Source: CAD feature listing. Evaluate the final solid. Frame: model axes, mm. Face numbers are marked on the shaded views. A direction names the side the tool comes from. Give positions to 0.01 mm unless a question says otherwise; leave off trailing zeros. Order: outer loops, then holes, each group sorted by start corner. A loop starts at its lowest first (then second) coordinate and runs counter-clockwise, first axis right, second up. Notation, with made-up numbers: M -35.75,-36 L 10.25,-36 A31 ccw 10.25,-3 Z; hole C -11,60 d8. An arc over 180 degrees is marked long. Answer as a JSON object with one key per item and string values. Group by question number.
1. Pull-direction query (Y, two-part tool) for the marked faces 1, 2, 3 and 4; classes: +Y half, -Y half, draft (parallel to the pull), parting line (faces both ways), or undercut.
2. Section query B-B (y = 75). Output: boundary loops of the cut face in (x, z) (3 decimals), plus the area to 3 significant figures.
3. Section query D-D (x = 20). Output: boundary loops of the cut face in (y, z).
4. Material intervals for L1, parallel to Y at x = 47, z = 4.1; L2, parallel to X at y = 18.5, z = 0.3; L3, parallel to Y at x = -2.5, z = 3.15, sorted ascending. Write a range as [from, to].
5. Section query A-A (x = 47). Output: boundary loops of the cut face in (y, z) (3 decimals), plus the area to 3 significant figures.
6. Set-up query: the marked faces 5 and 6. Return all of +Z, -Z, +X, -X, +Y, -Y with unobstructed straight access to the full face (end or side cutting, diameter ignored); none if empty.
7. Section query C-C (z = 5.1). Count the separate pieces of the cut face and the enclosed holes in it, plus the area to 3 significant figures.
8. Pin query (flat end, axial travel): P1, Ø1.8, axis at x = -3, y = 75, coming from the -Z side; P2, Ø3, axis at y = 66.5, z = 4, coming from the +X side; P3, Ø1.8, axis at x = -2.5, z = 4, coming from the -Y side. Return the tip coordinate at first contact, or that it passes through.
from build123d import *

# Parameters (mm, degrees)
BOSS_EXTRU_1_DEPTH       = 6
ESQUISSE2_R              = 1.5
ENL_V_MAT_EXTRU_1_DEPTH  = 6
ESQUISSE5_R              = 1.5
ENL_V_MAT_EXTRU_6_DEPTH  = 6
ESQUISSE6_R              = 2.995
ENL_V_MAT_EXTRU_7_DEPTH  = 3
ESQUISSE9_W              = 44
ESQUISSE9_H              = 20
BOSS_EXTRU_3_DEPTH       = 6
ESQUISSE10_W             = 25
ESQUISSE10_H             = 6.5
ENL_V_MAT_EXTRU_9_DEPTH  = 4
ENL_V_MAT_EXTRU_11_DEPTH = 6


with BuildPart() as part:
    # Esquisse1 → Boss.-Extru.1 (new body)
    with BuildSketch(Plane.XY):
        Polygon((0, 80), (0, 90), (44, 90), (44, 80), (50, 80), (50, 70), (44, 70), (44, 25), (50, 25), (50, 15), (44, 15), (44, 0), (0, 0), (0, 15), (-6, 15), (-6, 25), (0, 25), (0, 70), (-6, 70), (-6, 80), align=None)
    extrude(amount=BOSS_EXTRU_1_DEPTH)

    # Esquisse2 → Enlèv. mat.-Extru.1 (cut)
    with BuildSketch(Plane.XY.offset(6)):
        with Locations((20, 85)):
            Circle(ESQUISSE2_R)
    extrude(amount=-ENL_V_MAT_EXTRU_1_DEPTH, mode=Mode.SUBTRACT)

    # Esquisse5 → Enlèv. mat.-Extru.6 (cut)
    with BuildSketch(Plane(origin=(0, 0, 0), x_dir=(-1, 0, 0), z_dir=(0, 0, -1))):
        with Locations((3, 75)):
            Circle(ESQUISSE5_R)
        with Locations((3, 20)):
            Circle(ESQUISSE5_R)
        with Locations(Location((-47, 20, 0), (0, 0, 180))):
            Circle(ESQUISSE5_R)
        with Locations(Location((-47, 75, 0), (0, 0, 180))):
            Circle(ESQUISSE5_R)
    extrude(amount=-ENL_V_MAT_EXTRU_6_DEPTH, mode=Mode.SUBTRACT)

    # Esquisse6 → Enlèv. mat.-Extru.7 (cut)
    with BuildSketch(Plane(origin=(0, 0, 0), x_dir=(-1, 0, 0), z_dir=(0, 0, -1))):
        with Locations((3, 20)):
            Circle(ESQUISSE6_R)
        with Locations((3, 75)):
            Circle(ESQUISSE6_R)
        with Locations(Location((-47, 75, 0), (0, 0, 180))):
            Circle(ESQUISSE6_R)
        with Locations(Location((-47, 20, 0), (0, 0, 180))):
            Circle(ESQUISSE6_R)
    extrude(amount=-ENL_V_MAT_EXTRU_7_DEPTH, mode=Mode.SUBTRACT)

    # Esquisse9 → Boss.-Extru.3 (add)
    with BuildSketch(Plane.XY.offset(6)):
        with Locations((22, -10)):
            Rectangle(ESQUISSE9_W, ESQUISSE9_H)
    extrude(amount=-BOSS_EXTRU_3_DEPTH)

    # Esquisse10 → Enlèv. mat.-Extru.9 (cut)
    with BuildSketch(Plane.XY.offset(6)):
        with Locations((12.5, -9.75)):
            Rectangle(ESQUISSE10_W, ESQUISSE10_H)
    extrude(amount=-ENL_V_MAT_EXTRU_9_DEPTH, mode=Mode.SUBTRACT)

    # Esquisse11 → Enlèv. mat.-Extru.11 (cut)
    with BuildSketch(Plane.XY.offset(6)):
        Polygon((29, 71.292517007), (10, -2.207482993), (15, -3.5), (34, 70), align=None)
    extrude(amount=-ENL_V_MAT_EXTRU_11_DEPTH, mode=Mode.SUBTRACT)


solid = part.part
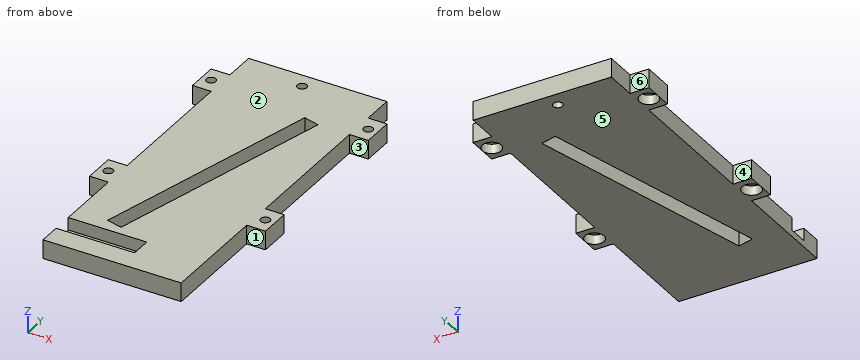
Answer sheet:
{
 "1": {"face 1": "-Y half", "face 2": "draft", "face 3": "undercut", "face 4": "undercut"},
 "2": {"outline": "M -6,0 L -5.995,0 L -5.995,3 L -4.5,3 L -4.5,6 L -6,6 Z; M -1.5,3 L -0.005,3 L -0.005,0 L 44.005,0 L 44.005,3 L 45.5,3 L 45.5,6 L -1.5,6 Z; M 48.5,3 L 49.995,3 L 49.995,0 L 50,0 L 50,6 L 48.5,6 Z", "area": "282 mm^2"},
 "3": {"outline": "M -20,0 L 15.84,0 L 15.84,6 L -6.5,6 L -6.5,2 L -13,2 L -13,6 L -20,6 Z; M 36.48,0 L 83.5,0 L 83.5,6 L 36.48,6 Z; M 86.5,0 L 90,0 L 90,6 L 86.5,6 Z"},
 "4": {"L1": "[15, 18.5], [21.5, 25], [70, 73.5], [76.5, 80]", "L2": "[-6, -5.59], [-0.41, 15.35], [20.69, 44.41], [49.59, 50]", "L3": "[15, 18.59], [21.41, 25], [70, 73.59], [76.41, 80]"},
 "5": {"outline": "M 15,0 L 17.005,0 L 17.005,3 L 18.5,3 L 18.5,6 L 15,6 Z; M 21.5,3 L 22.995,3 L 22.995,0 L 25,0 L 25,6 L 21.5,6 Z; M 70,0 L 72.005,0 L 72.005,3 L 73.5,3 L 73.5,6 L 70,6 Z; M 76.5,3 L 77.995,3 L 77.995,0 L 80,0 L 80,6 L 76.5,6 Z", "area": "66.1 mm^2"},
 "6": {"face 5": "-Z, +X, -X, +Y, -Y", "face 6": "+Z, -Z, -X, +Y"},
 "7": {"separate pieces": "1", "enclosed holes": "6", "area": "4,490 mm^2"},
 "8": {"P1": "through", "P2": "x = 44", "P3": "y = 15"}
}
